```python
from build123d import *

# Parameters (mm, degrees)
SKETCH1_W           = 42.9449992
SKETCH1_H           = 29.972
BOSS_EXTRUDE1_DEPTH = 1.524
SKETCH2_R           = 3.175
BOSS_EXTRUDE2_DEPTH = 1.524
SKETCH3_R           = 1.143
CUT_EXTRUDE1_DEPTH  = 56.024518955
FILLET1_R           = 3.175


with BuildPart() as part:
    # Sketch1 → Boss-Extrude1 (new body)
    with BuildSketch(Plane.XY):
        with Locations((21.4724996, 14.986)):
            Rectangle(SKETCH1_W, SKETCH1_H)
    extrude(amount=BOSS_EXTRUDE1_DEPTH)

    # Sketch2 → Boss-Extrude2 (add)
    with BuildSketch(Plane.XY.offset(1.524)):
        with Locations((0, 14.986)):
            Circle(SKETCH2_R)
        with Locations((42.9449992, 14.986)):
            Circle(SKETCH2_R)
    extrude(amount=-BOSS_EXTRUDE2_DEPTH)

    # Sketch3 → Cut-Extrude1 (cut, through all)
    with BuildSketch(Plane.XY.offset(1.524)):
        with Locations((0, 14.986)):
            Circle(SKETCH3_R)
        with Locations((42.9449992, 14.986)):
            Circle(SKETCH3_R)
    extrude(amount=-CUT_EXTRUDE1_DEPTH, mode=Mode.SUBTRACT)

    # Fillet1
    fillet1_edges = [part.edges().sort_by_distance(p)[0] for p in [
        (0, 29.972, 0.762),
        (42.9449992, 29.972, 0.762),
        (42.9449992, 0, 0.762),
        (0, 0, 0.762),
    ]]
    fillet(fillet1_edges, radius=FILLET1_R)


solid = part.part
```
Could you check a few things on this model? Use its own coordinates, in mm. A direction names the side the tool comes from. Give positions to 0.01 mm unless a question says otherwise; leave off trailing zeros. Order: outer loops, then holes, each group sorted by start corner. A loop starts at its lowest first (then second) coordinate and runs counter-clockwise, first axis right, second up.
Q1. For faces 1 (the flat face through (0, 7, 1)), 2 (the flat face through (42.945, 22, 1)), 3 (the flat face through (42.945, 7, 1)), 4 (the cylindrical face through (0.91, 29.02, 0.77)), which set-ups out of +Z, -Z, +X, -X, +Y, -Y let a thin tool reach every point of the face, with its end or its side?
Q2. If I drill on line 1 along X through (y, z) = (26, 1.4) (3 decimals); line 2 along Y through (x, z) = (-0.5, 1.1); line 3 along X through (y, z) = (27.5, 0.35), over which ranges is the centre line in solid material (lowest first)?
Q3. Suppose I cut it at A-A, the plane z = 1.05. Write out the boundary of the cut face in (x, y) (3 decimals), and give its area (3 significant figures).
Q4. Suppose I cut it at B-B, the plane y = 19.5. Write out the boundary of the cut face in (x, z) (3 decimals), and give its area (3 significant figures).
Q5. Suppose I cut it at C-C, the plane x = 2. Write out the boundary of the cut face in (y, z).
Q6. We'd pull the mould along X, two halves only. Please class faces 5 (the flat face through (0, 22, 1)), 6 (the flat face through (21, 0, 1)), 7 (the cylindrical face through (42.103, 15.758, 0.773)): +X half, -X half, draft (parallel to the pull), parting line (faces both ways), or undercut.
Q7. I'm going to push flat-ended pins straight in: P1, Ø0.8, axis at y = 24, z = 1, coming from the +X side (3 decimals); P2, Ø0.8, axis at y = 6.5, z = 0.5, coming from the -X side. Where does each tip first touch, or does it pass through?
Solution:
1. face 1: +Z, -Z, -X, -Y
1. face 2: +Z, -Z, +X, +Y
1. face 3: +Z, -Z, +X, -Y
1. face 4: +Z, -Z, -X, +Y
2. line 1: x = 0 to 42.945
2. line 2: y = 11.85 to 13.96, 16.01 to 18.12
2. line 3: x = 0.08 to 42.87
3. outline: (0, 3.175) arc R3.175 ccw to (3.175, 0) - (39.77, 0) arc R3.175 ccw to (42.945, 3.175) - (42.945, 11.811) arc R3.175 ccw to (42.945, 18.161) - (42.945, 26.797) arc R3.175 ccw to (39.77, 29.972) - (3.175, 29.972) arc R3.175 ccw to (0, 26.797) - (0, 18.161) arc R3.175 ccw to (0, 11.811) - close; hole circle Ø2.286 at (0, 14.986); hole circle Ø2.286 at (42.945, 14.986)
3. area: 1,300 mm2
4. outline: (0, 0) - (42.945, 0) - (42.945, 1.524) - (0, 1.524) - close
4. area: 65.4 mm2
5. outline: (0.23, 0) - (29.75, 0) - (29.75, 1.52) - (0.23, 1.52) - close
6. face 5: -X half
6. face 6: draft
6. face 7: undercut
7. P1: stops at x = 42.945
7. P2: stops at x = 0
